```python
from build123d import *

# Parameters (mm, degrees)
SKETCH1_W           = 57.4
SKETCH1_H           = 41.4
SKETCH1_W_2         = 25.4
SKETCH1_H_2         = 25.4
BOSS_EXTRUDE1_DEPTH = 30
SKETCH2_W           = 57.4
SKETCH2_H           = 41.4
BOSS_EXTRUDE2_DEPTH = 10
BOSS_EXTRUDE3_DEPTH = 8
BOSS_EXTRUDE4_START = -8
BOSS_EXTRUDE4_DEPTH = 8
CUT_EXTRUDE1_REACH  = 104.774
SKETCH6_R           = 2.5
CUT_EXTRUDE4_REACH  = 104.774
SKETCH9_R           = 2.5
SKETCH7_R           = 4
CUT_EXTRUDE2_DEPTH  = 2
CUT_EXTRUDE3_START  = -2
SKETCH8_R           = 4
CUT_EXTRUDE3_DEPTH  = 2


with BuildPart() as part:
    # Sketch1 → Boss-Extrude1 (new body)
    with BuildSketch(Plane.XY):
        Rectangle(SKETCH1_W, SKETCH1_H)
        Rectangle(SKETCH1_W_2, SKETCH1_H_2, mode=Mode.SUBTRACT)
    extrude(amount=BOSS_EXTRUDE1_DEPTH)

    # Sketch2 → Boss-Extrude2 (add)
    with BuildSketch(Plane.XY.offset(30)):
        Rectangle(SKETCH2_W, SKETCH2_H)
    extrude(amount=BOSS_EXTRUDE2_DEPTH)

    # Sketch4 → Boss-Extrude3 (add)
    with BuildSketch(Plane(origin=(28.7, 0, 0), x_dir=(0, 0, -1), z_dir=(1, 0, 0))):
        with BuildLine():
            Line((-40, -20.7), (-40, 20.7))
            Line((-40, 20.7), (-62, 20.7))
            ThreePointArc((-62, 20.7), (-82.7, 0), (-62, -20.7))
            Line((-62, -20.7), (-40, -20.7))
        make_face()
    extrude(amount=-BOSS_EXTRUDE3_DEPTH)

    # Sketch5 → Boss-Extrude4 (add)
    with BuildSketch(Plane.ZY.offset(28.7).offset(BOSS_EXTRUDE4_START)):
        with BuildLine():
            Line((40, 20.7), (40, -20.7))
            Line((40, -20.7), (62, -20.7))
            ThreePointArc((62, -20.7), (82.7, 0), (62, 20.7))
            Line((62, 20.7), (40, 20.7))
        make_face()
    extrude(amount=BOSS_EXTRUDE4_DEPTH)

    # Cut-Extrude1: up to this face of the body (flat: up to its plane)
    cut_extrude1_end = Plane(part.part.faces().sort_by_distance((-28.7, 0, 39.26525255))[0])
    # Sketch6 → Cut-Extrude1 (cut, up to the picked face)
    with BuildSketch(Plane(origin=(28.7, 0, 0), x_dir=(0, 0, -1), z_dir=(1, 0, 0)), mode=Mode.PRIVATE) as cut_extrude1_sk1:
        with Locations((-62, 0)):
            Circle(SKETCH6_R)
    cut_extrude1_tool1 = split(extrude(cut_extrude1_sk1.sketch, amount=-CUT_EXTRUDE1_REACH, mode=Mode.PRIVATE), bisect_by=cut_extrude1_end, keep=Keep.BOTH, mode=Mode.PRIVATE)
    add(cut_extrude1_tool1.solids().sort_by(Axis((28.7, 0, 62), (-1, 0, 0)))[0], mode=Mode.SUBTRACT)

    # Cut-Extrude4: up to this face of the body (flat: up to its plane)
    cut_extrude4_end = Plane(part.part.faces().sort_by_distance((-28.7, 0, 39.126630479))[0])
    # Sketch9 → Cut-Extrude4 (cut, up to the picked face)
    with BuildSketch(Plane(origin=(28.7, 0, 0), x_dir=(0, 0, -1), z_dir=(1, 0, 0)), mode=Mode.PRIVATE) as cut_extrude4_sk1:
        with Locations((-12.5, 0)):
            Circle(SKETCH9_R)
    cut_extrude4_tool1 = split(extrude(cut_extrude4_sk1.sketch, amount=-CUT_EXTRUDE4_REACH, mode=Mode.PRIVATE), bisect_by=cut_extrude4_end, keep=Keep.BOTH, mode=Mode.PRIVATE)
    add(cut_extrude4_tool1.solids().sort_by(Axis((28.7, 0, 12.5), (-1, 0, 0)))[0], mode=Mode.SUBTRACT)

    # Sketch7 → Cut-Extrude2 (cut)
    with BuildSketch(Plane.ZY.offset(28.7)):
        with Locations((62, 0)):
            Circle(SKETCH7_R)
        with Locations((12.5, 0)):
            Circle(SKETCH7_R)
    extrude(amount=-CUT_EXTRUDE2_DEPTH, mode=Mode.SUBTRACT)

    # Sketch8 → Cut-Extrude3 (cut)
    with BuildSketch(Plane(origin=(28.7, 0, 0), x_dir=(0, 0, -1), z_dir=(1, 0, 0)).offset(CUT_EXTRUDE3_START)):
        with Locations(Location((-62, 0, 0), (0, 0, 180))):
            Circle(SKETCH8_R)
        with Locations(Location((-12.5, 0, 0), (0, 0, 180))):
            Circle(SKETCH8_R)
    extrude(amount=CUT_EXTRUDE3_DEPTH, mode=Mode.SUBTRACT)


solid = part.part
```
Design review of the part built by this model. Coordinates are the model's own, in mm. A direction names the side the tool comes from. Round coordinates to 2 decimals unless told otherwise and drop trailing zeros. Write each loop counter-clockwise with the first axis right and the second up, starting at its lowest first coordinate (ties: lowest second). Pieces come first, ordered by that corner, then holes. Notation, with made-up numbers: (28.5, -36.5) -> (44.5, -36.5) arc R9 cw to (44.5, -31.5) -> close; hole circle Ø5 at (46.5, 76.5). An arc over 180 degrees is marked (long way). Write item = value, one per line. Start each with the question number.
1) Clearance check with flat-ended pins moving along their axes: pin 1 (4.5 mm diameter, centred on y = 0, z = 62, fed in from -X); pin 2 (4 mm diameter, centred on y = 0, z = 60.5, fed in from -X); pin 3 (12.5 mm diameter, centred on x = 1.5, y = -1, fed in from +Z); pin 4 (6.5 mm diameter, centred on y = 0, z = 12.5, fed in from +X). State where each tip first meets the part, or that it passes through.
2) Mouldability with a two-part tool opening along Z and no side actions: class faces 5 (the face through (0, 0, 30)), 6 (the face through (27.686, 1.532, 65.695)), 7 (the face through (0, -20.7, 24)) as +Z half, -Z half, draft (parallel to the pull), parting line (faces both ways), or undercut.
3) Take a section at B-B, the plane z = 23. State the section outline as (x, y) points.
4) Take a section at A-A, the plane z = 12.5. State the section outline as (x, y) points, plus the area to 3 significant figures.
5) Take a section at C-C, the plane x = -3. State the section outline as (y, z) points.
6) Wall thickness on probe 1 along X at (y, z) = (-3, 9); probe 2 along Y at (x, z) = (-5, 12); probe 3 along X at (y, z) = (5, 63): over which ranges is each line inside the solid? List them lowest first. Write a range as from..to.
7) Tool access review of faces 1 (the face through (20.7, 0, 57)), 2 (the face through (0, -12.7, 15)), 3 (the face through (26.7, 3, 12)), 4 (the face through (-27.714, -1.532, 65.695)): name each direction out of +Z, -Z, +X, -X, +Y, -Y from which nothing blocks a thin tool from reaching the whole face with its end or side.
8) Take a section at D-D, the plane x = -15. State the section outline as (y, z) points.
Results list:
q1.pin_1 = through
q1.pin_2 = -26.7
q1.pin_3 = 40
q1.pin_4 = 26.7
q2.face_5 = -Z half
q2.face_6 = undercut
q2.face_7 = draft
q3.outline = (-28.7, -20.7) -> (28.7, -20.7) -> (28.7, 20.7) -> (-28.7, 20.7) -> close; hole (-12.7, -12.7) -> (12.7, -12.7) -> (12.7, 12.7) -> (-12.7, 12.7) -> close
q4.outline = (-28.7, -20.7) -> (28.7, -20.7) -> (28.7, -4) -> (26.7, -4) -> (26.7, -2.5) -> (12.7, -2.5) -> (12.7, -12.7) -> (-12.7, -12.7) -> (-12.7, -2.5) -> (-26.7, -2.5) -> (-26.7, -4) -> (-28.7, -4) -> close; (-28.7, 4) -> (-26.7, 4) -> (-26.7, 2.5) -> (-12.7, 2.5) -> (-12.7, 12.7) -> (12.7, 12.7) -> (12.7, 2.5) -> (26.7, 2.5) -> (26.7, 4) -> (28.7, 4) -> (28.7, 20.7) -> (-28.7, 20.7) -> close
q4.area = 1,560 mm²
q5.outline = (-20.7, 0) -> (-12.7, 0) -> (-12.7, 30) -> (12.7, 30) -> (12.7, 0) -> (20.7, 0) -> (20.7, 40) -> (-20.7, 40) -> close
q6.probe_1 = -28.7..-12.7, 12.7..28.7
q6.probe_2 = -20.7..-12.7, 12.7..20.7
q6.probe_3 = -28.7..-20.7, 20.7..28.7
q7.face_1 = +Z, +Y, -Y
q7.face_2 = -Z
q7.face_3 = +X
q7.face_4 = -X
q8.outline = (-20.7, 0) -> (20.7, 0) -> (20.7, 40) -> (-20.7, 40) -> close; hole circle Ø5 at (0, 12.5)
